Work out the finished part from the listing and answer in its coordinate system (mm). A direction names the side the tool comes from. Round coordinates to 2 decimals unless told otherwise and drop trailing zeros. Order: outer loops, then holes, each group sorted by start corner. A loop starts at its lowest first (then second) coordinate and runs counter-clockwise, first axis right, second up. Notation, with made-up numbers: M -32,24.5 L 15,24.5 A24 cw 15,60.5 Z; hole C 86,-16 d10. An arc over 180 degrees is marked long. Return JSON: item names as keys, results as strings.
from build123d import *

# Parameters (mm, degrees)
F1_DEPTH = 4
F2_T     = 0.5
F3_R     = 0.25


# Not quite as in the source:
# - a shell that OpenCascade refuses in one call is made with other operations: the cavity is built on its own and cut out


with BuildPart() as f1:
    # F0 (on Top) → F1 (new body)
    with BuildSketch(Plane.XY):
        with BuildLine():
            Line((10.5, 10.835), (-10.5, 10.835))
            ThreePointArc((-10.5, 10.835), (-10.8535533906, 10.6885533906), (-11, 10.335))
            Line((-11, 10.335), (-11, -10.335))
            ThreePointArc((-11, -10.335), (-10.8535533906, -10.6885533906), (-10.5, -10.835))
            Line((-10.5, -10.835), (10.5, -10.835))
            ThreePointArc((10.5, -10.835), (10.8535533906, -10.6885533906), (11, -10.335))
            Line((11, -10.335), (11, 10.335))
            ThreePointArc((11, 10.335), (10.8535533906, 10.6885533906), (10.5, 10.835))
        make_face()
    extrude(amount=F1_DEPTH)

    # F2: shell of thickness 0.5, made by hand


with BuildPart() as f2_core1:
    # F2_t2: copy of F1
    add(f1.part)

    # the walls: a layer under each face that stays
    f2_faces = [f2_core1.faces().sort_by_distance(p)[0] for p in [
        (0, 10.835, 2),
        (-11, 0, 2),
        (0, -10.835, 2),
        (11, 0, 2),
        (0, 0, 0),
    ]]
    thicken(f2_faces, amount=-F2_T, mode=Mode.SUBTRACT)


with BuildPart() as f1_1:
    add(f1.part)

    # what is left inside the walls is the cavity
    f2_cavity = [f2_core1.part.solids().sort_by_distance(p)[0] for p in [
        (0, -3.445, 0.505),
    ]]
    add(f2_cavity, mode=Mode.SUBTRACT)

    # F3
    f3_edges = [f1_1.edges().sort_by_distance(p)[0] for p in [
        (10.5, 0, 4),
        (0, 10.335, 4),
        (-10.5, 0, 4),
        (0, -10.335, 4),
    ]]
    fillet(f3_edges, radius=F3_R)


solid = f1_1.part
Item 1: Consider line 1 along X through (y, z) = (-0.25, 2.2); line 2 along Y through (x, z) = (6.5, 2) (3 decimals); line 3 along Z through (x, y) = (-6.5, 7.5). Determine where each line is inside the solid, lowest interval first. Write a range as [from, to].
Output:
{"line 1": "x = [-11, -10.5], [10.5, 11]", "line 2": "y = [-10.835, -10.335], [10.335, 10.835]", "line 3": "z = [0, 0.5]"}
Item 2: Find section A-A (z = 1.6). Determine the outline of the cut face in (x, y) (3 decimals), plus the area to 3 significant figures.
Output:
{"outline": "M -11,-10.335 A0.5 ccw -10.5,-10.835 L 10.5,-10.835 A0.5 ccw 11,-10.335 L 11,10.335 A0.5 ccw 10.5,10.835 L -10.5,10.835 A0.5 ccw -11,10.335 Z; hole M -10.5,-10.335 L 10.5,-10.335 L 10.5,10.335 L -10.5,10.335 Z", "area": "42.5 mm^2"}
Item 3: The mould has two halves that part along Y. Classify faces 1 (the flat face through (0, 0, 0)), 2 (the flat face through (0, 0, 0.5)), 3 (the flat face through (10.5, 0, 2)), 4 (the flat face through (0, 10.835, 2)): pulls with the +Y half, pulls with the -Y half, needs draft (parallel to the pull), parting line crosses it, or undercut.
Output:
{"face 1": "needs draft", "face 2": "undercut", "face 3": "undercut", "face 4": "pulls with the +Y half"}
Item 4: Find section C-C (y = 0.25). Determine the outline of the cut face in (x, z).
Output:
{"outline": "M -11,0 L 11,0 L 11,4 L 10.75,4 A0.25 ccw 10.5,3.75 L 10.5,0.5 L -10.5,0.5 L -10.5,3.75 A0.25 ccw -10.75,4 L -11,4 Z"}
Item 5: Which of the six approach directions +Z, -Z, +X, -X, +Y, -Y give full straight-line access (tool end or side, diameter ignored) to faces 5 (the flat face through (0, -10.335, 2)), 6 (the flat face through (0, -10.835, 2))?
Output:
{"face 5": "+Z", "face 6": "+Z, -Z, +X, -X, -Y"}
Item 6: Find section B-B (x = 9). Determine the outline of the cut face in (y, z) (3 decimals), plus the area to 3 significant figures.
Output:
{"outline": "M -10.835,0 L 10.835,0 L 10.835,4 L 10.585,4 A0.25 ccw 10.335,3.75 L 10.335,0.5 L -10.335,0.5 L -10.335,3.75 A0.25 ccw -10.585,4 L -10.835,4 Z", "area": "14.3 mm^2"}
